from build123d import *

# Parameters (mm, degrees)
SKETCH1_W           = 20
SKETCH1_H           = 20
BOSS_EXTRUDE1_DEPTH = 20
SKETCH1_4_R         = 2.5
BOSS_EXTRUDE3_DEPTH = 10
SKETCH5_W           = 2.4
SKETCH5_H           = 1.8
CUT_EXTRUDE1_DEPTH  = 6.2
SKETCH8_R           = 2.5
BOSS_EXTRUDE4_DEPTH = 10
SKETCH10_W          = 20
SKETCH10_H          = 20
BOSS_EXTRUDE5_DEPTH = 40
BOSS_EXTRUDE5_TAPER = 10


with BuildPart() as part:
    # Sketch1 → Boss-Extrude1 (new body)
    with BuildSketch(Plane(origin=(0, 0, 0), x_dir=(1, 0, 0), z_dir=(0, 1, 0))):
        with Locations((10, -10)):
            Rectangle(SKETCH1_W, SKETCH1_H)
    extrude(amount=BOSS_EXTRUDE1_DEPTH)

    # Sketch1<4> → Boss-Extrude3 (add)
    with BuildSketch(Plane(origin=(0, 0, 0), x_dir=(1, 0, 0), z_dir=(0, 1, 0))):
        Polygon((13, 0), (7, 0), (7, -1.8), (4.6, -1.8), (4.6, -3.6), (7, -6.1), (13, -6.1), (15.4, -3.6), (15.4, -1.8), (13, -1.8), align=None)
        Polygon((0, -7), (0, -13), (1.8, -13), (1.8, -15.4), (3.6, -15.4), (6.1, -13), (6.1, -7), (3.6, -4.6), (1.8, -4.6), (1.8, -7), align=None)
        Polygon((20, -7), (18.2, -7), (18.2, -4.6), (16.4, -4.6), (13.9, -7), (13.9, -13), (16.4, -15.4), (18.2, -15.4), (18.2, -13), (20, -13), align=None)
        with Locations(Location((10, -10, 0), (0, 0, 270))):
            Circle(SKETCH1_4_R)
    extrude(amount=-BOSS_EXTRUDE3_DEPTH)

    # Sketch5 → Cut-Extrude1 (cut)
    with BuildSketch(Plane.XY.offset(20)):
        with Locations((14.3, 0.9)):
            Rectangle(SKETCH5_W, SKETCH5_H)
        with Locations((5.7, 0.9)):
            Rectangle(SKETCH5_W, SKETCH5_H)
        Polygon((6.9, 6.1), (4.5, 3.6), (4.5, 1.8), (6.9, 1.8), (6.9, 0), (13.1, 0), (13.1, 1.8), (15.5, 1.8), (15.5, 3.6), (13.1, 6.1), align=None)
        Polygon((4.5, 5.364), (4.5, 3.6), (6.9, 6.1), (5.266666667, 6.1), align=None)
        Polygon((14.733333333, 6.1), (13.1, 6.1), (15.5, 3.6), (15.5, 5.364), align=None)
        Polygon((15.5, 6.1), (14.733333333, 6.1), (15.5, 5.364), align=None)
        Polygon((4.5, 6.1), (4.5, 5.364), (5.266666667, 6.1), align=None)
    extrude(amount=-CUT_EXTRUDE1_DEPTH, mode=Mode.SUBTRACT)

    # Sketch8 → Boss-Extrude4 (add)
    with BuildSketch(Plane.XY.offset(20)):
        Polygon((13, 20), (7, 20), (7, 18.2), (4.6, 18.2), (4.6, 16.4), (7, 13.9), (13, 13.9), (15.4, 16.4), (15.4, 18.2), (13, 18.2), align=None)
        Polygon((0, 13), (0, 7), (1.8, 7), (1.8, 4.6), (3.6, 4.6), (4.5, 5.464), (4.5, 6.1), (5.1625, 6.1), (6.1, 7), (6.1, 13), (3.6, 15.4), (1.8, 15.4), (1.8, 13), align=None)
        Polygon((20, 13), (18.2, 13), (18.2, 15.4), (16.4, 15.4), (13.9, 13), (13.9, 7), (14.8375, 6.1), (15.5, 6.1), (15.5, 5.464), (16.4, 4.6), (18.2, 4.6), (18.2, 7), (20, 7), align=None)
        with Locations(Location((10, 10, 0), (0, 0, 180))):
            Circle(SKETCH8_R)
    extrude(amount=BOSS_EXTRUDE4_DEPTH)

    # Sketch10 → Boss-Extrude5 (add)
    with BuildSketch(Plane.ZY):
        with Locations((10, 10)):
            Rectangle(SKETCH10_W, SKETCH10_H)
    extrude(amount=BOSS_EXTRUDE5_DEPTH, taper=BOSS_EXTRUDE5_TAPER)


solid = part.part
The listing builds one solid part. Answer for the finished solid, in the listing's coordinates (mm). A direction names the side the tool comes from. Coordinates: 2 decimals unless noted, no trailing zeros. Loops run counter-clockwise (first coordinate to the right, second up) from the corner with the lowest first, then second, coordinate; pieces in that order, holes last. Notation, with made-up numbers: M 31.5,65 L 68.5,65 A17 ccw 68.5,69 Z; hole C 81,47.5 d8. An arc over 180 degrees is marked long. Answer in a Markdown table with one row per item.
1) Given pin 1 (0.9 mm diameter, centred on x = 1, y = -6, fed in from -Z); pin 2 (2 mm diameter, centred on x = 1, z = 25, fed in from -Y); pin 3 (1.4 mm diameter, centred on y = 17.5, z = 23, fed in from +X), each flat-ended and moving along its own axis, determine where each tip first touches the part or whether it passes through.
Answers below:
| item | result |
|---|---|
| pin 1 | z = 7 |
| pin 2 | y = 4.6 |
| pin 3 | x = 15.4 |
2) Find section B-B (x = 10). Determine the outline of the cut face in (y, z).
Answers below:
| item | result |
|---|---|
| outline | M -10,0 L 20,0 L 20,30 L 13.9,30 L 13.9,20 L 12.5,20 L 12.5,30 L 7.5,30 L 7.5,20 L 6.1,20 L 6.1,13.8 L 0,13.8 L 0,12.5 L -10,12.5 L -10,7.5 L 0,7.5 L 0,6.1 L -10,6.1 Z |
3) Determine the mould class of faces 1 (the cylindrical face through (7.56, -4.93, 9.46)), 2 (the flat face through (17, 10, 30)), 3 (the flat face through (7, -5, 1)) for opening direction Z: released by +Z, released by -Z, zero draft, split by the parting line, or undercut.
Answers below:
| item | result |
|---|---|
| face 1 | undercut |
| face 2 | released by +Z |
| face 3 | zero draft |
4) Find the intervals of material crossed by probe 1 along Z at (x, y) = (14, 14.5); probe 2 along Y at (x, z) = (10, 26); probe 3 along X at (y, z) = (14.5, 23), in increasing order.
Answers below:
| item | result |
|---|---|
| probe 1 | 0 to 20 |
| probe 2 | 7.5 to 12.5, 13.9 to 20 |
| probe 3 | 1.8 to 4.54, 6.42 to 13.58, 15.46 to 18.2 |
5) Find section A-A (y = -4.5). Count the separate pieces of the cut face and the enclosed holes in it, then the cut area to 3 significant figures.
Answers below:
| item | result |
|---|---|
| separate pieces | 4 |
| enclosed holes | 0 |
| area | 173 mm^2 |
6) Which of the six approach directions +Z, -Z, +X, -X, +Y, -Y give full straight-line access (tool end or side, diameter ignored) to faces 4 (the flat face through (14.18, 15.13, 24.93)), 5 (the flat face through (5.78, -4.93, 4.83)), 6 (the flat face through (18.2, -5, 6))?
Answers below:
| item | result |
|---|---|
| face 4 | +Z |
| face 5 | -Y |
| face 6 | -Z, +X, -Y |
